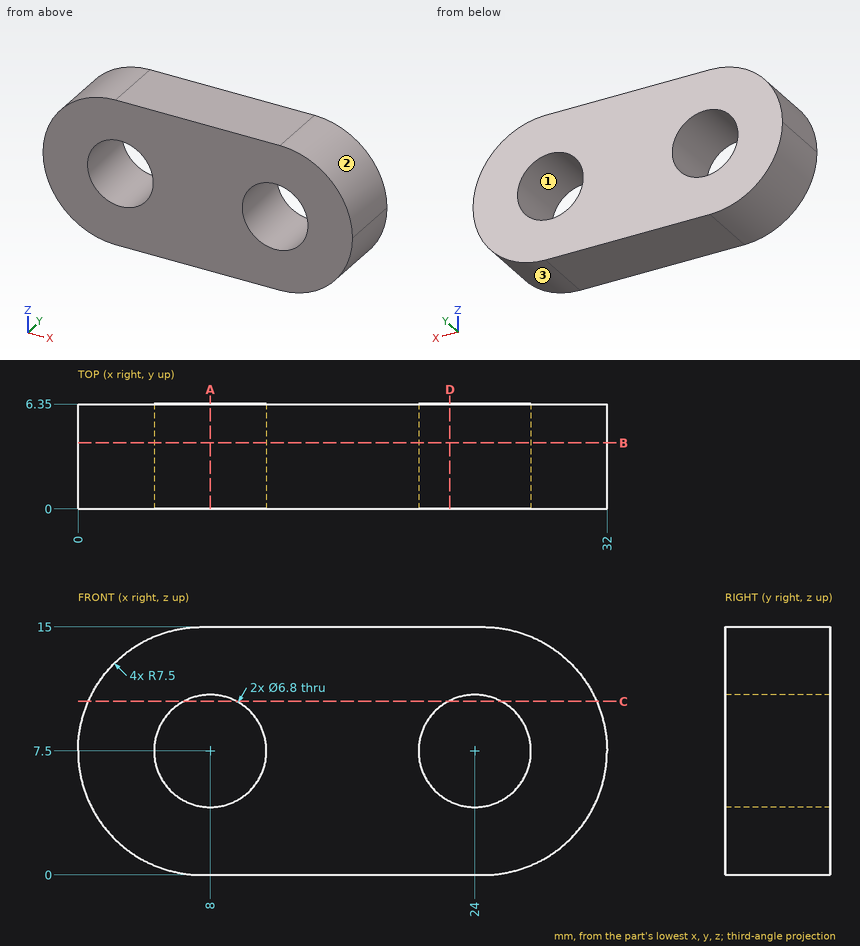
Drawing for the job (mm, zero at the part's lowest x, y, z). Give positions to 0.01 mm unless a question says otherwise; leave off trailing zeros. Loops run counter-clockwise (first coordinate to the right, second up) from the corner with the lowest first, then second, coordinate; pieces in that order, holes last.
1) Band-saw the part on C-C on z = 10.5. List the corners of the cut face in (x, y).
Values follow:
outline: (0.63, 0) - (6.4, 0) - (6.4, 6.35) - (0.63, 6.35) - close; (9.6, 0) - (22.4, 0) - (22.4, 6.35) - (9.6, 6.35) - close; (25.6, 0) - (31.37, 0) - (31.37, 6.35) - (25.6, 6.35) - close
2) Band-saw the part on B-B on y = 4. State how many separate pieces and enclosed holes the cut face has, then the cut area to 3 significant figures.
Values follow:
separate pieces: 1
enclosed holes: 2
area: 359 mm2
3) Band-saw the part on A-A on x = 8. List the corners of the cut face in (y, z), then the cut area to 3 significant figures.
Values follow:
outline: (0, 0) - (6.35, 0) - (6.35, 4.1) - (0, 4.1) - close; (0, 10.9) - (6.35, 10.9) - (6.35, 15) - (0, 15) - close
area: 52.1 mm2
4) Drop flat-ended pins along their axis: P1, Ø1, axis at y = 4, z = 8.5, coming from the -X side; P2, Ø1.5, axis at y = 3, z = 3, coming from the -X side (1 decimal). Give the stop position or say it passes through.
Values follow:
P1: stops at x = 0.02
P2: stops at x = 1
5) Band-saw the part on D-D on x = 22.5. List the corners of the cut face in (y, z).
Values follow:
outline: (0, 0) - (6.35, 0) - (6.35, 4.45) - (0, 4.45) - close; (0, 10.55) - (6.35, 10.55) - (6.35, 15) - (0, 15) - close
6) Two-plate mould, pull along Z, no slides. Class the marked faces 1, 2 and 3: released by +Z, released by -Z, zero draft, split by the parting line, or undercut.
Values follow:
face 1: undercut
face 2: released by +Z
face 3: released by -Z
7) Probe line 1 along X through (y, z) = (2.5, 7.5); line 2 along Z through (x, y) = (24.5, 4.75); line 3 along Z through (x, y) = (5.5, 5.75). List the from-to ranges inside material, lowest first.
Values follow:
line 1: x = 0 to 4.6, 11.4 to 20.6, 27.4 to 32
line 2: z = 0 to 4.14, 10.86 to 15
line 3: z = 0.27 to 5.2, 9.8 to 14.73
